For this review, take the finished solid that the model builds, in its own axes (mm). Face numbers are marked on the shaded views. Coordinates: 2 decimals unless noted, no trailing zeros. Loops run counter-clockwise (first coordinate to the right, second up) from the corner with the lowest first, then second, coordinate; pieces in that order, holes last. Notation, with made-up numbers: (-18, 6) -> (-7, 6) arc R26 ccw to (-7, 43) -> close; hole circle Ø6 at (65.25, 29). An arc over 180 degrees is marked (long way). Answer in a Markdown table with one row per item.
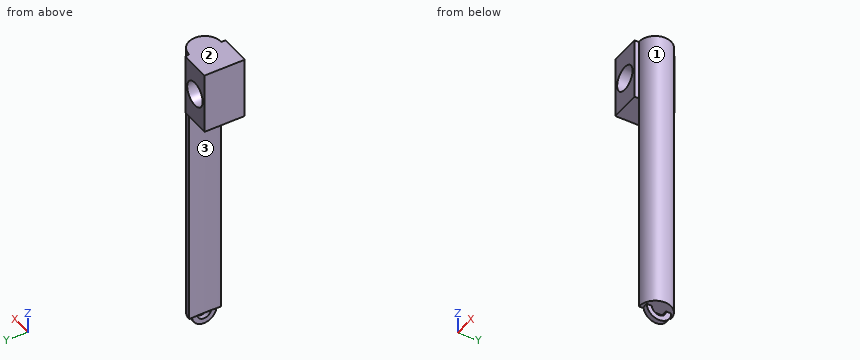
from build123d import *

# Parameters (mm, degrees)
F1_DEPTH  = 59.69
F3_DEPTH  = 12.7
F5_R      = 2.54
F6_DEPTH  = 25.4
F8_DEPTH  = 52.07
F9_W      = 75.692
F9_H      = 5.588
F10_DEPTH = 25.4


with BuildPart() as f1:
    # F0 (on Top) → F1 (new body)
    with BuildSketch(Plane.XY):
        with BuildLine():
            ThreePointArc((50.692685, 3.300256), (50.8, 0), (50.692685, -3.300256))
            ThreePointArc((50.692685, -3.300256), (54.102, 0), (50.692685, 3.300256))
        make_face()
    extrude(amount=F1_DEPTH)

    # F2 (on face) → F3 (join)
    with BuildSketch(Plane.XY.offset(59.69)):
        with BuildLine():
            Line((44.27921, -4.162097), (50.62921, -4.162097))
            ThreePointArc((50.62921, -4.162097), (50.8, 0), (50.62921, 4.162097))
            Line((50.62921, 4.162097), (44.27921, 4.162097))
            Line((44.27921, 4.162097), (44.27921, -4.162097))
        make_face()
    extrude(amount=-F3_DEPTH)

    # F5 (on face) → F6 (cut)
    with BuildSketch(Plane(origin=(0, 4.162097, 0), x_dir=(-1, 0, 0), z_dir=(0, 1, 0))):
        with Locations((-47.445018, 53.337224)):
            Circle(F5_R)
    extrude(amount=-F6_DEPTH, mode=Mode.SUBTRACT)

    # F7 (on Right) → F8 (join)
    with BuildSketch(Plane.YZ):
        with BuildLine():
            ThreePointArc((1.46637, 0), (0, -1.46637), (-1.46637, 0))
            Line((-1.46637, 0), (-2.54, 0))
            ThreePointArc((-2.54, 0), (0, -2.54), (2.54, 0))
            Line((2.54, 0), (1.46637, 0))
        make_face()
    extrude(amount=F8_DEPTH)

    # F9 (on Top) → F10 (cut)
    with BuildSketch(Plane.XY):
        with Locations((13.186903, 0.036883)):
            Rectangle(F9_W, F9_H)
    extrude(amount=-F10_DEPTH, mode=Mode.SUBTRACT)


solid = f1.part
Item 1: Take a section at B-B, the plane x = 46. State the section outline as (y, z) points.
Worked answers:
| item | result |
|---|---|
| outline | (-4.16, 46.99) -> (4.16, 46.99) -> (4.16, 51.25) -> (-4.16, 51.25) -> close; (-4.16, 55.43) -> (4.16, 55.43) -> (4.16, 59.69) -> (-4.16, 59.69) -> close |
Item 2: The part is to be moulded in two halves that separate along Y. For the marked faces 1, 2 and 3, say which applies: +Y half, -Y half, draft (parallel to the pull), parting line (faces both ways), or undercut.
Worked answers:
| item | result |
|---|---|
| face 1 | parting line |
| face 2 | draft |
| face 3 | undercut |
Item 3: Take a section at D-D, the plane x = 48.75. State the section outline as (y, z) points, and give its area (3 significant figures).
Worked answers:
| item | result |
|---|---|
| outline | (-4.16, 46.99) -> (4.16, 46.99) -> (4.16, 51.16) -> (-4.16, 51.16) -> close; (-4.16, 55.52) -> (4.16, 55.52) -> (4.16, 59.69) -> (-4.16, 59.69) -> close |
| area | 69.4 mm² |
Item 4: Take a section at A-A, the plane y = -0.25. State the section outline as (x, z) points.
Worked answers:
| item | result |
|---|---|
| outline | (44.28, 46.99) -> (50.8, 46.99) -> (50.8, 0) -> (54.09, 0) -> (54.09, 59.69) -> (44.28, 59.69) -> close; (51.03, -2.53) -> (52.07, -2.53) -> (52.07, -1.44) -> (51.03, -1.44) -> close; hole circle Ø5.08 at (47.45, 53.34) |
Item 5: Insertion check: pin 1 (1.5 mm diameter, centred on x = 46.5, y = 2.5, fed in from -Z); pin 2 (0.8 mm diameter, centred on y = -1, z = -1, fed in from -X); pin 3 (1.3 mm diameter, centred on y = 0, z = -2, fed in from +X). Each pin has a flat end and moves straight along its axis. Give the tip position at first contact, or say it passes through.
Worked answers:
| item | result |
|---|---|
| pin 1 | z = 46.99 |
| pin 2 | x = 51.03 |
| pin 3 | x = 52.07 |
Item 6: For L1, parallel to Z at x = 50.5, y = 2.5; L2, parallel to Z at x = 46.75, y = 1; L3, parallel to X at y = 0, z = 30, list the stretches that pass through material, from the lowest coordinate up.
Worked answers:
| item | result |
|---|---|
| L1 | 46.99 to 59.69 |
| L2 | 46.99 to 50.89, 55.78 to 59.69 |
| L3 | 50.8 to 54.1 |
